For this review, use the dimensioned drawing (mm, ordinates from the lowest corner) and the shaded views. A direction names the side the tool comes from. Coordinates: 2 decimals unless noted, no trailing zeros. Write each loop counter-clockwise with the first axis right and the second up, starting at its lowest first coordinate (ties: lowest second). Pieces come first, ordered by that corner, then holes. Notation, with made-up numbers: (72.5, 76) - (91.5, 76) arc R10 ccw to (91.5, 93) - close; hole circle Ø1 at (-26.75, 35.25). An arc over 180 degrees is marked (long way). Answer as a JSON object with one key per item and string values.
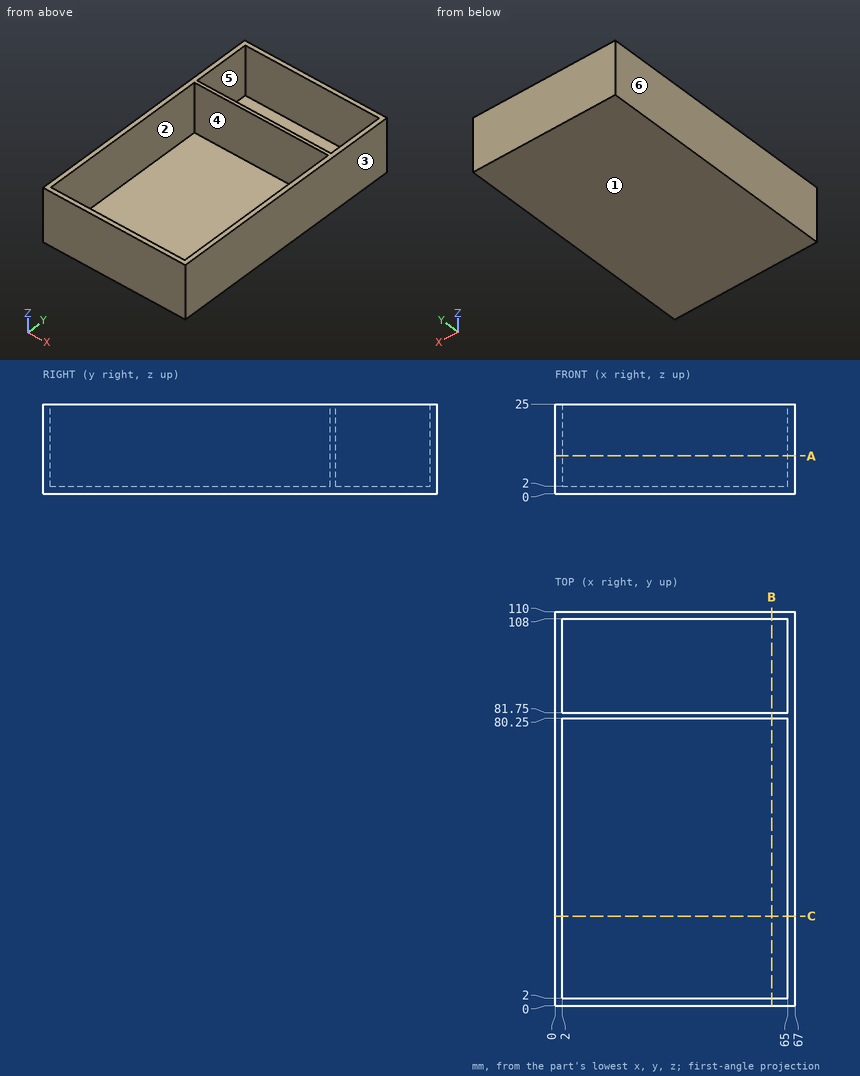
(1) The part is to be moulded in two halves that separate along X. For the marked faces 3, 4, 5 and 6, say which applies: pulls with the +X half, pulls with the -X half, needs draft (parallel to the pull), parting line crosses it, or undercut.
Solved:
{"face 3": "pulls with the +X half", "face 4": "undercut", "face 5": "undercut", "face 6": "pulls with the -X half"}
(2) Take a section at A-A, the plane z = 10.5. Write out the cut boundary in (x, y), and give its area (4 significant figures).
Solved:
{"outline": "(0, 0) - (67, 0) - (67, 110) - (0, 110) - close; hole (2, 2) - (65, 2) - (65, 80.25) - (2, 80.25) - close; hole (2, 81.75) - (65, 81.75) - (65, 108) - (2, 108) - close", "area": "786.5 mm^2"}
(3) Tool access review of the marked faces 1 and 2: name each direction out of +Z, -Z, +X, -X, +Y, -Y from which nothing blocks a thin tool from reaching the whole face with its end or side.
Solved:
{"face 1": "-Z, +X, -X, +Y, -Y", "face 2": "+Z"}
(4) To check wall thickness, follow line 1 (Y direction, x = 22, z = 7.5); line 2 (X direction, y = 100.5, z = 12.25); line 3 (Z direction, x = 21.5, y = 74). State the ranges of each line that lie inside material, in increasing order. Write a range as from..to.
Solved:
{"line 1": "y = 0..2, 80.25..81.75, 108..110", "line 2": "x = 0..2, 65..67", "line 3": "z = 0..2"}
(5) Take a section at B-B, the plane x = 60.5. Write out the cut boundary in (y, z), and give its area (4 significant figures).
Solved:
{"outline": "(0, 0) - (110, 0) - (110, 25) - (108, 25) - (108, 2) - (81.75, 2) - (81.75, 25) - (80.25, 25) - (80.25, 2) - (2, 2) - (2, 25) - (0, 25) - close", "area": "346.5 mm^2"}
(6) For pin 1 (8 mm diameter, centred on x = 47.5, y = 49, fed in from +Z), flat-tipped, find the tip position at first contact; note if it passes through.
Solved:
{"pin 1": "stops at z = 2"}
(7) Take a section at C-C, the plane y = 25. Write out the cut boundary in (x, z), and give its area (3 significant figures).
Solved:
{"outline": "(0, 0) - (67, 0) - (67, 25) - (65, 25) - (65, 2) - (2, 2) - (2, 25) - (0, 25) - close", "area": "226 mm^2"}
